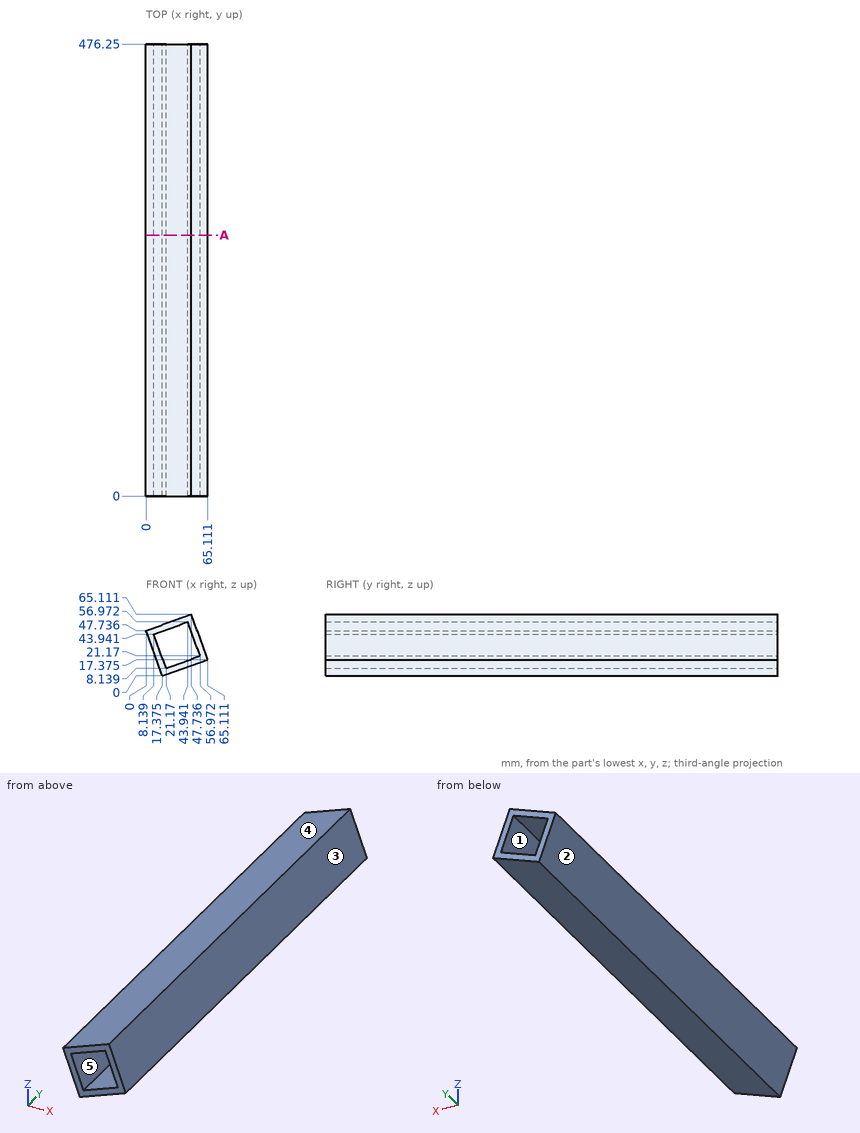
Drawing for the job (mm, zero at the part's lowest x, y, z). A direction names the side the tool comes from. Round coordinates to 2 decimals unless told otherwise and drop trailing zeros. Order: outer loops, then holes, each group sorted by start corner. A loop starts at its lowest first (then second) coordinate and runs counter-clockwise, first axis right, second up.
Item 1: Tool access for the marked faces 1 and 2: list every direction of +Z, -Z, +X, -X, +Y, -Y with a clear straight run to the whole face (end or side of a thin tool).
Item 2: Saw through at A-A on y = 275. Write the cut outline in (x, z) (1 decimal), then the cut area to 3 significant figures.
Item 3: Pin check, flat tips, straight feed: pin 1 (8 mm diameter, centred on y = 158.5, z = 28.5, fed in from +X); pin 2 (4 mm diameter, centred on x = 52.5, z = 24.5, fed in from -Y); pin 3 (6 mm diameter, centred on x = 18.5, y = 193.5, fed in from +Z); pin 4 (5 mm diameter, centred on x = 31.5, y = 168.5, fed in from +Z). Stop position of each tip, or through.
Item 4: Probe line 1 along X through (y, z) = (384, 28) (1 decimal); line 2 along X through (y, z) = (36, 35) (1 decimal); line 3 along Z through (x, y) = (40, 371) (1 decimal). List the from-to ranges inside material, lowest first.
Item 5: Mould opens along X. For the marked faces 3, 4 and 5 say: pulls with the +X half, pulls with the -X half, needs draft (parallel to the pull), parting line crosses it, or undercut.
Reported:
1. face 1: +Y, -Y
1. face 2: -Z, -X, +Y, -Y
2. outline: (0, 47.7) - (17.4, 0) - (65.1, 17.4) - (47.7, 65.1) - close; hole (8.1, 43.9) - (21.2, 8.1) - (57, 21.2) - (43.9, 57) - close
2. area: 1,130 mm2
3. pin 1: stops at x = 62.52
3. pin 2: passes through
3. pin 3: stops at z = 55.56
3. pin 4: stops at z = 60.11
4. line 1: x = 7.2 to 13.9, 54.5 to 61.2
4. line 2: x = 4.6 to 11.4, 51.9 to 58.7
4. line 3: z = 8.2 to 15, 55.5 to 62.3
5. face 3: pulls with the +X half
5. face 4: pulls with the -X half
5. face 5: undercut
